Autodesk Inventor part; units mm, degrees
ref_plane "YZ Plane" through (0, 0, 0) normal (1, 0, 0) x (0, 1, 0)
ref_plane "XZ Plane" through (0, 0, 0) normal (0, 1, 0) x (-1, 0, 0)
ref_plane "XY Plane" through (0, 0, 0) normal (0, 0, 1) x (1, 0, 0)
sketch "Sketch1" plane through (0, 0, 0) normal (0, 0, 1) x (1, 0, 0)
  line L0 (0, -4) -> (0, -20)
  line L1 (4, 0) -> (26, 0)
  line L2 (26, 3) -> (-3, 3)
  line L3 (-3, 3) -> (-3, -20)
  line L4 (26, 3) -> (26, 0)
  line L5 (0, -20) -> (-3, -20)
  line L6 (4, 0) -> (0, -4)
  point P0 (0, 0)
  point P1 (0, 0)
  dimension "d0" = 20
  dimension "d1" = 26
  dimension "d2" = 3
  dimension "d5" = 4
  dimension "d6" = 4
extrude "Extrusion1" add sketch "Sketch1" along normal blind 30
sketch "Sketch2" plane through (-3, 3, 0) normal (0, 1, 0) x (1, 0, 0)
  line L0 (29, 0) -> (0, 0)
  line L1 (29, 0) -> (29, -30)
  point P0 (3, 0)
  point P1 (24, -6)
  point P2 (24, -15.2)
  dimension "d9" = 9.2
  dimension "d10" = 6
  dimension "d11" = 5
  dimension "d12" = 5
hole "Hole1" at (21, 3, 6) at (21, 3, 15.2) direction (0, -1, 0) diameter 1 end through all
sketch "Sketch3" plane through (0, -20, 0) normal (1, 0, 0) x (0, 0, -1)
  line L0 (0, 0) -> (0, 16)
  line L1 (0, 0) -> (-30, 0)
  line L2 (0, 16) -> (-30, 16)
  point P0 (0, 20)
  point P1 (-3.5, 10.5)
  point P2 (-26.5, 4.5)
  dimension "d20" = 3.5
  dimension "d29" = 5.5
  dimension "d30" = 23
  dimension "d31" = 6
hole "Hole2" at (0, -9.5, 3.5) at (0, -15.5, 26.5) direction (-1, 0, 0) diameter 4 end through all
properties part number "Estrutura - SensorX"
Could you check a few things on this model? Use its own coordinates, in mm. A direction names the side the tool comes from. Give positions to 0.01 mm unless a question says otherwise; leave off trailing zeros. Order: outer loops, then holes, each group sorted by start corner. A loop starts at its lowest first (then second) coordinate and runs counter-clockwise, first axis right, second up. Notation, with made-up numbers: (52.5, 45) - (100.5, 45) arc R28 cw to (100.5, 76) - close; hole circle Ø11 at (83, 0). An arc over 180 degrees is marked (long way). Return JSON: item names as keys, results as strings. Group by question number.
Q1. Suppose I cut it at A-A, the plane z = 3.5. Please give me the cut outline in (x, y), and give its area (3 significant figures).
Q2. Suppose I cut it at D-D, the plane z = 11.5. Please give me the cut outline in (x, y).
Q3. Thinking about a two-plate mould opening in X: for faces 1 (the face through (20.504, 1.479, 5.935)), 2 (the face through (2, -2, 15)), 3 (the face through (6, 1, 0)), which applies, pulls with the +X half, pulls with the -X half, needs draft (parallel to the pull), parting line crosses it, or undercut?
Q4. Which directions (+Z, -Z, +X, -X, +Y, -Y) give clear straight access to the entire face, cutting with the end or side of a thin tool? Please do faces 4 (the face through (15, 0, 15)), 5 (the face through (-1.521, -17.186, 25.425)).
Q5. Suppose I cut it at C-C, the plane y = -9.5. Please give me the cut outline in (x, z), and give its area (3 significant figures).
Q6. Will these pins go through, and if not, where does the flat tip stop? pin 1 Ø3 at (y, z) = (-15.5, 26.5) entering from -X; pin 2 Ø4 at (x, z) = (17.5, 11) entering from -Y; pin 3 Ø1 at (y, z) = (-5, 25) entering from +X; pin 4 Ø6 at (x, z) = (4, 16.5) entering from -Y.
Q7. Suppose I cut it at B-B, the plane x = 21. Please give me the cut outline in (y, z).
Q8. Please list where these lines run through material, in increasing order: line 1 along X through (y, z) = (1.6, 6); line 2 along Y through (x, z) = (-1.7, 26.5); line 3 along X through (y, z) = (-16.25, 9.5). Write a range as [from, to].
Resolved:
{
 "1": {"outline": "(-3, -20) - (0, -20) - (0, -11.5) - (-3, -11.5) - close; (-3, -7.5) - (0, -7.5) - (0, -4) - (4, 0) - (26, 0) - (26, 3) - (-3, 3) - close", "area": "143 mm2"},
 "2": {"outline": "(-3, -20) - (0, -20) - (0, -4) - (4, 0) - (26, 0) - (26, 3) - (-3, 3) - close"},
 "3": {"face 1": "undercut", "face 2": "pulls with the +X half", "face 3": "needs draft"},
 "4": {"face 4": "+Z, -Z, +X, -Y", "face 5": "+X, -X"},
 "5": {"outline": "(-3, 0) - (0, 0) - (0, 1.5) - (-3, 1.5) - close; (-3, 5.5) - (0, 5.5) - (0, 30) - (-3, 30) - close", "area": "78.0 mm2"},
 "6": {"pin 1": "passes through", "pin 2": "stops at y = 0", "pin 3": "stops at x = 0", "pin 4": "stops at y = -3"},
 "7": {"outline": "(0, 0) - (3, 0) - (3, 5.5) - (0, 5.5) - close; (0, 6.5) - (3, 6.5) - (3, 14.7) - (0, 14.7) - close; (0, 15.7) - (3, 15.7) - (3, 30) - (0, 30) - close"},
 "8": {"line 1": "x = [-3, 20.5], [21.5, 26]", "line 2": "y = [-20, -17.5], [-13.5, 3]", "line 3": "x = [-3, 0]"}
}
